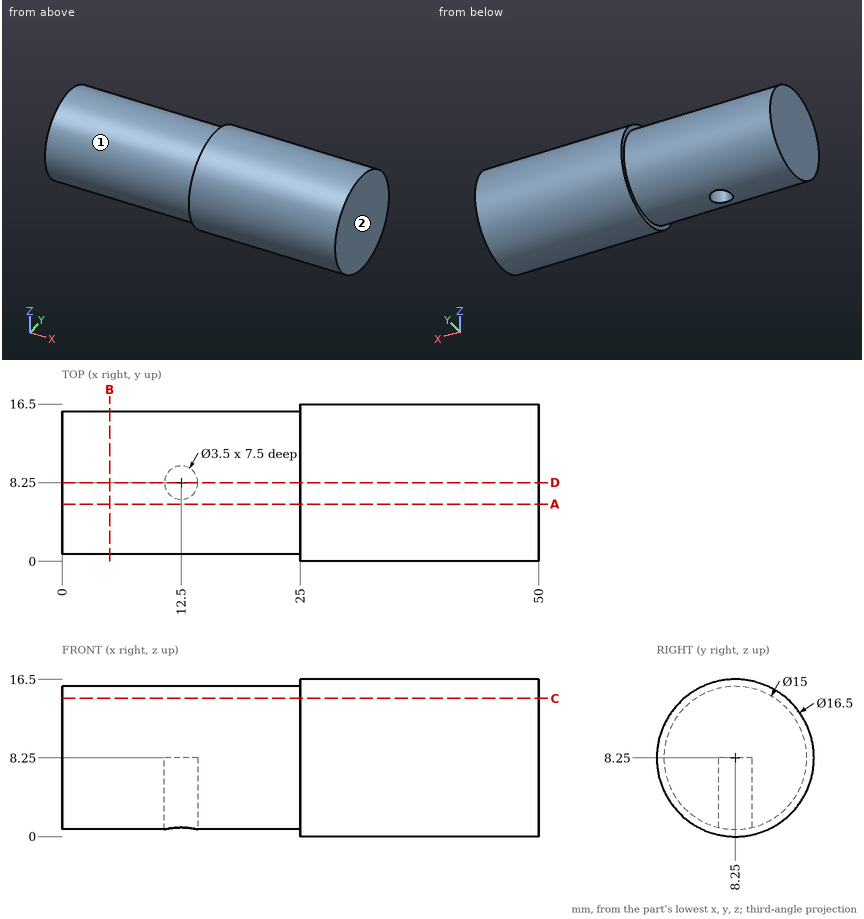
For this review, use the dimensioned drawing (mm, ordinates from the lowest corner) and the shaded views. A direction names the side the tool comes from. Give positions to 0.01 mm unless a question says otherwise; leave off trailing zeros. Order: outer loops, then holes, each group sorted by start corner. A loop starts at its lowest first (then second) coordinate and runs counter-clockwise, first axis right, second up.
1. To check wall thickness, follow L1, parallel to X at y = 8.25, z = 3.5; L2, parallel to X at y = 8.75, z = 1; L3, parallel to Y at x = 12.5, z = 6.75. State the ranges of each line that lie inside material, in increasing order.
Solution:
L1: x = 0 to 10.75, 14.25 to 50
L2: x = 0 to 10.82, 14.18 to 50
L3: y = 0.9 to 6.5, 10 to 15.6
2. Add section A-A, the plane y = 6. State the section outline as (x, z) points, then the cut area to 3 significant figures.
Solution:
outline: (0, 1.1) - (25, 1.1) - (25, 0.31) - (50, 0.31) - (50, 16.19) - (25, 16.19) - (25, 15.4) - (0, 15.4) - close
area: 755 mm2
3. Add section B-B, the plane x = 5. State the section outline as (y, z) points.
Solution:
outline: circle Ø15 at (8.25, 8.25)
4. For pin 1 Ø6 at (x, z) = (33, 2.5) entering from +Y; pin 2 Ø1 at (x, z) = (43, 8.5) entering from -Y; pin 3 Ø2 at (x, y) = (12.5, 8.25) entering from +Z; pin 4 Ø6 at (x, y) = (33.5, 4) entering from -Z, all flat-tipped, find the tip position at first contact; note any pin that passes through.
Solution:
pin 1: stops at y = 16.03
pin 2: stops at y = 0
pin 3: stops at z = 15.75
pin 4: stops at z = 0.1
5. Tool access review of the marked faces 1 and 2: name each direction out of +Z, -Z, +X, -X, +Y, -Y from which nothing blocks a thin tool from reaching the whole face with its end or side.
Solution:
face 1: -X
face 2: +Z, -Z, +X, +Y, -Y
6. Add section C-C, the plane z = 14.5. State the section outline as (x, y) points, then the cut area to 3 significant figures.
Solution:
outline: (0, 4.1) - (25, 4.1) - (25, 2.86) - (50, 2.86) - (50, 13.64) - (25, 13.64) - (25, 12.4) - (0, 12.4) - close
area: 477 mm2
7. Add section D-D, the plane y = 8.25. State the section outline as (x, z) points, then the cut area to 3 significant figures.
Solution:
outline: (0, 0.75) - (10.75, 0.75) - (10.75, 8.25) - (14.25, 8.25) - (14.25, 0.75) - (25, 0.75) - (25, 0) - (50, 0) - (50, 16.5) - (25, 16.5) - (25, 15.75) - (0, 15.75) - close
area: 761 mm2
